Read the model definition and answer for the solid it produces. Units are mm, in the model's axes. A direction names the side the tool comes from. Coordinates: 2 decimals unless noted, no trailing zeros. Write each loop counter-clockwise with the first axis right and the second up, starting at its lowest first coordinate (ties: lowest second). Pieces come first, ordered by that corner, then holes.
Item 1: Section A-A (x = 0) is taken. Give the vertices of the cut face in (y, z), then the cut area to 3 significant figures.
Item 2: Straight lines are drawn through the part: probe 1 along Y at (x, z) = (0, 7); probe 2 along Z at (x, y) = (-8.25, -2.5); probe 3 along Y at (x, z) = (-3.25, 5). For each, find the intervals that lie inside material, in ascending order.
Item 3: Determine the mould class of faces 3 (the face through (-0.59, 4.46, 5.45)), 4 (the face through (-4.42, 1.54, 9)), 5 (the face through (4.38, -8.43, 0.99)) for opening direction Y: released by +Y, released by -Y, zero draft, split by the parting line, or undercut.
Item 4: Section D-D (y = 8) is taken. Give the vertices of the cut face in (x, z), then the cut area to 3 significant figures.
Item 5: Section C-C (z = 7.5) is taken. Give the vertices of the cut face in (x, y), then the cut area to 3 significant figures.
Item 6: Each of these flat-tipped pins is pushed along its axis until it touches: P1, Ø1, axis at x = 6.5, z = 7.5, coming from the +Y side; P2, Ø1.5, axis at x = -2, z = 4.5, coming from the +Y side; P3, Ø2.5, axis at x = 0.5, y = 1.5, coming from the +Z side. Where does it stop, or does it pass through?
Item 7: A tool of negligible diameter and unlimited length cuts with its end or side. For faces 1 (the face through (0, 0, 2)), 2 (the face through (0, 0, 0)), from which of +Z, -Z, +X, -X, +Y, -Y can it reach the whole face along a straight path? Write none if from no direction.
from build123d import *

# Parameters (mm, degrees)
F0_R     = 9.5
F0_R_2   = 6.5
F1_DEPTH = 2
F0_R_3   = 4.5
F2_DEPTH = 9
F3_DEPTH = 2


with BuildPart() as f1:
    # F0 (on Top) → F1 (new body)
    with BuildSketch(Plane.XY):
        Circle(F0_R)
        Circle(F0_R_2, mode=Mode.SUBTRACT)
    extrude(amount=F1_DEPTH)

    # F0 (on Top) → F2 (join)
    with BuildSketch(Plane.XY):
        Circle(F0_R_2)
        Circle(F0_R_3, mode=Mode.SUBTRACT)
    extrude(amount=F2_DEPTH)

    # F0 (on Top) → F3 (join)
    with BuildSketch(Plane.XY):
        Circle(F0_R_3)
    extrude(amount=F3_DEPTH)


solid = f1.part
Established:
1. outline: (-9.5, 0) - (9.5, 0) - (9.5, 2) - (6.5, 2) - (6.5, 9) - (4.5, 9) - (4.5, 2) - (-4.5, 2) - (-4.5, 9) - (-6.5, 9) - (-6.5, 2) - (-9.5, 2) - close
1. area: 66.0 mm2
2. probe 1: y = -6.5 to -4.5, 4.5 to 6.5
2. probe 2: z = 0 to 2
2. probe 3: y = -5.63 to -3.11, 3.11 to 5.63
3. face 3: undercut
3. face 4: zero draft
3. face 5: split by the parting line
4. outline: (-5.12, 0) - (5.12, 0) - (5.12, 2) - (-5.12, 2) - close
4. area: 20.5 mm2
5. outline: circle Ø13 at (0, 0); hole circle Ø9 at (0, 0)
5. area: 69.1 mm2
6. P1: stops at y = 2.5
6. P2: stops at y = 6.38
6. P3: stops at z = 2
7. face 1: +Z
7. face 2: -Z, +X, -X, +Y, -Y
